Geometry check sheet. Reference: the model listing, model coordinates, mm. Face numbers are marked on the shaded views. Round coordinates to 2 decimals unless told otherwise and drop trailing zeros. Loops run counter-clockwise (first coordinate to the right, second up) from the corner with the lowest first, then second, coordinate; pieces in that order, holes last. Notation, with made-up numbers: (39, 81.5) - (51, 81.5) arc R12 cw to (51, 100.5) - close; hole circle Ø5 at (28, 65). An arc over 180 degrees is marked (long way). Write item = value, one per line.
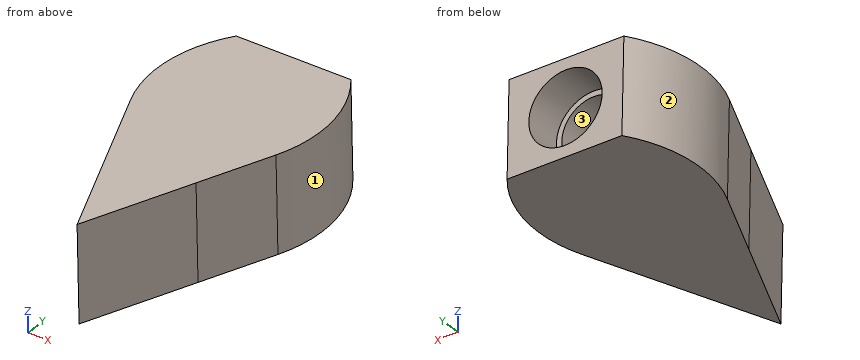
```python
from build123d import *

# Parameters (mm, degrees)
BOSS_EXTRUDE1_DEPTH      = 4.35
BOSS_EXTRUDE1_DEPTH_BACK = 3.2
SKETCH4_R                = 2.45
CUT_EXTRUDE2_DEPTH       = 10
SKETCH4_5_R              = 2.875
SKETCH4_5_R_2            = 2.45
CUT_EXTRUDE3_DEPTH       = 3
FILLET1_R                = 10
BOSS_EXTRUDE2_DEPTH      = 7.55


with BuildPart() as part:
    # Sketch2 → Boss-Extrude1 (new, two sides: drawn at the far end of the back side and taken through both)
    with BuildSketch(Plane(origin=(0, 0.021487422, -0.580480419), x_dir=(1, 0, 0), z_dir=(0, -0.02843310858496513, 0.9995956974378171)).offset(-BOSS_EXTRUDE1_DEPTH_BACK)):
        Polygon((-13.116179094, 1.214943373), (-10.360421829, -5.408768885), (-2.99346614, -23.115914326), (3.822823349, -23.115914326), (11.189779038, -5.408768885), (13.945536303, 1.214943373), (9.430107454, -3.300485476), (4.914678604, -7.815914326), (-4.085321396, -7.815914326), (-8.600750245, -3.300485476), align=None)
    extrude(amount=BOSS_EXTRUDE1_DEPTH + BOSS_EXTRUDE1_DEPTH_BACK)

    # Sketch4 → Cut-Extrude2 (cut)
    with BuildSketch(Plane(origin=(0, -7.80778247, -0.222089318), x_dir=(1, 0, 0), z_dir=(0, 0.9995956974378171, 0.02843310858496514))):
        with Locations(Location((0.414678604, 0.005856684, 0), (0, 0, 270))):
            Circle(SKETCH4_R)
    extrude(amount=-CUT_EXTRUDE2_DEPTH, mode=Mode.SUBTRACT)

    # Sketch4<5> → Cut-Extrude3 (cut)
    with BuildSketch(Plane(origin=(0, -7.80778247, -0.222089318), x_dir=(1, 0, 0), z_dir=(0, 0.9995956974378171, 0.02843310858496514))):
        with Locations(Location((0.414678604, 0.005856684, 0), (0, 0, 270))):
            Circle(SKETCH4_5_R)
        with Locations(Location((0.414678604, 0.005856684, 0), (0, 0, 270))):
            Circle(SKETCH4_5_R_2, mode=Mode.SUBTRACT)
    extrude(amount=-CUT_EXTRUDE3_DEPTH, mode=Mode.SUBTRACT)

    # Fillet1
    # the kernel refuses this fillet: 10 mm, written as the material it takes off along each edge
    with BuildSketch(Plane(origin=(13.945536303, -0.3371442, 54.757471627), x_dir=(-0.7071067811865475, -0.7068208961031768, -0.020105243890642274), z_dir=(0, 0.028433108584965117, -0.999595697437817)), Plane(origin=(-13.116179094, 2.776325306, -54.69980818), x_dir=(0.7071067811865489, -0.7068208961031754, -0.020105243890642235), z_dir=(0, -0.028433108584965117, 0.999595697437817))) as fillet1_piece_1:
        with BuildLine():
            CenterArc((22.662755022, 1.47115243), FILLET1_R, 188.459787479, 59.129683347)
            Line((18.850352296, -7.773607462), (0, 0))
            Line((0, 0), (12.771561437, 0))
        make_face()
    extrude(amount=109.501551565, mode=Mode.SUBTRACT)

    # Sketch6 → Boss-Extrude2 (add)
    with BuildSketch(Plane(origin=(0, -0.107168461, 3.767619442), x_dir=(1, 0, 0), z_dir=(0, -0.02843310858496513, 0.9995956974378171))):
        Polygon((-2.99346614, -23.110940453), (0.414678604, -31.302725123), (3.822823349, -23.110940453), align=None)
    extrude(amount=-BOSS_EXTRUDE2_DEPTH)


solid = part.part
```
(1) Section check C-C (x = -1.75). Enter the section's corners in (y, z).
Answers follow:
outline = (-26.2, 3.03) - (-25.98, -4.52) - (-7.7, -4) - (-7.75, -2.12) - (-10.75, -2.2) - (-10.77, -1.46) - (-17.77, -1.66) - (-17.84, 0.63) - (-10.84, 0.83) - (-10.86, 1.58) - (-7.86, 1.66) - (-7.91, 3.55) - close
(2) Section check D-D (x = 4.25). Enter the section's corners in (y, z), then the cut area to 3 significant figures.
Answers follow:
outline = (-22.18, 3.14) - (-21.97, -4.41) - (-7.7, -4) - (-7.91, 3.55) - close
area = 108 mm²
(3) Gauge pin test, flat ends, axial feed: pin 1 (1 mm diameter, centred on x = 3, z = -1.5, fed in from -Y); pin 2 (1.5 mm diameter, centred on y = -23, z = -1, fed in from -X). Record the tip position at first contact, or that the pin passes through.
Answers follow:
pin_1 = -26.26
pin_2 = -3.34
(4) Section check B-B (y = -28.5). Enter the section's corners in (x, z), then the cut area to 3 significant figures.
Answers follow:
outline = (-0.79, 2.96) - (-0.7, -4.59) - (1.53, -4.59) - (1.62, 2.96) - close
area = 17.5 mm²
(5) Mould release check, pull along X, two halves, no side actions. Record for the marked faces 1, 2 and 3: pulls with the +X half, pulls with the -X half, needs draft (parallel to the pull), parting line crosses it, or undercut.
Answers follow:
face_1 = pulls with the +X half
face_2 = pulls with the -X half
face_3 = undercut
(6) Scan lines: L1, parallel to Z at x = -1.75, y = -9; L2, parallel to Z at x = -0.25, y = -14.25; L3, parallel to Y at x = 4.5, z = 2.75. Record each from-to range of solid material in increasing order. Write a range as [from, to].
Answers follow:
L1 = [-4.04, -2.15], [1.63, 3.51]
L2 = [-4.19, -2.77], [1.95, 3.37]
L3 = [-21.57, -7.89]
(7) Section check A-A (x = 1). Enter the section's corners in (y, z), then the cut area to 3 significant figures.
Answers follow:
outline = (-29.99, 2.92) - (-29.78, -4.63) - (-7.7, -4) - (-7.73, -3.04) - (-10.73, -3.13) - (-10.74, -2.69) - (-17.74, -2.89) - (-17.87, 1.87) - (-10.87, 2.06) - (-10.89, 2.5) - (-7.89, 2.59) - (-7.91, 3.55) - close
area = 117 mm²
